from build123d import *

# Parameters (mm, degrees)
F0_R      = 19.05
F1_DEPTH  = 101.6
F2_R      = 16.672802
F3_DEPTH  = 101.6
F5_DEPTH  = 101.6
F7_DEPTH  = 101.6
F9_DEPTH  = 101.6
F11_DEPTH = 101.6


with BuildPart() as f1:
    # F0 (on Right) → F1 (new body)
    with BuildSketch(Plane.YZ):
        Circle(F0_R)
    extrude(amount=F1_DEPTH)

    # F2 (on face) → F3 (cut)
    with BuildSketch(Plane.YZ.offset(101.6)):
        Circle(F2_R)
    extrude(amount=-F3_DEPTH, mode=Mode.SUBTRACT)

    # F4 (on face) → F5 (join)
    with BuildSketch(Plane(origin=(0, 0, 0), x_dir=(0, -1, 0), z_dir=(-1, 0, 0))):
        with BuildLine():
            Line((0, 19.05), (2.557494, 18.877545))
            ThreePointArc((2.557494, 18.877545), (5.998328, 44.666261), (2.622403, 70.463553))
            Line((2.622403, 70.463553), (0, 70.597149))
            ThreePointArc((0, 70.597149), (4.50405, 44.823575), (0, 19.05))
        make_face()
    extrude(amount=-F5_DEPTH)

    # F6 (on face) → F7 (join)
    with BuildSketch(Plane.YZ.offset(101.6)):
        with BuildLine():
            Line((-1.23902, -71.141139), (1.281651, -71.141139))
            ThreePointArc((1.281651, -71.141139), (5.279028, -45.073988), (1.281651, -19.006837))
            Line((1.281651, -19.006837), (-1.612408, -18.98164))
            ThreePointArc((-1.612408, -18.98164), (3.484779, -45.026237), (-1.23902, -71.141139))
        make_face()
    extrude(amount=-F7_DEPTH)

    # F8 (on face) → F9 (join)
    with BuildSketch(Plane(origin=(0, 0, 0), x_dir=(0, -1, 0), z_dir=(-1, 0, 0))):
        with BuildLine():
            Line((18.974914, 0), (18.974914, -1.689716))
            ThreePointArc((18.974914, -1.689716), (45.881311, -5.978723), (72.88587, -2.358837))
            Line((72.88587, -2.358837), (72.733122, -0.475401))
            ThreePointArc((72.733122, -0.475401), (45.817013, -4.422211), (18.974914, 0))
        make_face()
    extrude(amount=-F9_DEPTH)

    # F10 (on face) → F11 (join)
    with BuildSketch(Plane.YZ.offset(101.6)):
        with BuildLine():
            ThreePointArc((19.039206, -0.641189), (45.322797, 2.394132), (71.440637, -1.836555))
            Line((71.440637, -1.836555), (71.576953, 0.641189))
            ThreePointArc((71.576953, 0.641189), (45.30808, 4.934439), (19.039206, 0.641189))
            Line((19.039206, 0.641189), (19.039206, -0.641189))
        make_face()
    extrude(amount=-F11_DEPTH)


solid = f1.part
Read the model definition and answer for the solid it produces. Units are mm, in the model's axes. Give positions to 0.01 mm unless a question says otherwise; leave off trailing zeros. Write each loop counter-clockwise with the first axis right and the second up, starting at its lowest first coordinate (ties: lowest second). Pieces come first, ordered by that corner, then holes. Notation, with made-up numbers: (28.25, 37) - (54.25, 37) arc R20 cw to (54.25, 50) - close; hole circle Ø2 at (28.5, 89.5). An arc over 180 degrees is marked (long way). Answer in a Markdown table with one row per item. Add a question column.
Item 1: Flat-ended cylindrical pins translate along their axes: P1, Ø4, axis at x = 23, y = 43.5, coming from the +Z side; P2, Ø4, axis at x = 90, y = 19.5, coming from the -Z side; P3, Ø1, axis at x = 61, z = 42.5, coming from the +Y side; P4, Ø20, axis at y = 0, z = 0, coming from the -X side. Find the tip coordinate at first contact, or state that the pin passes through.
Item 2: Determine the mould class of faces 1 (the face through (51.5, 45, 2.4)), 2 (the face through (101.6, -6, -16)), 3 (the face through (51.51, 3.48, -44.65)) for opening direction Z: pulls with the +Z half, pulls with the -Z half, needs draft (parallel to the pull), parting line crosses it, or undercut.
Item 3: Section B-B, the plane z = 42 is taken. Write down the section's boundary in (x, y).
Item 4: Section A-A, the plane x = 38 is taken. Write down the section's boundary in (y, z).
Item 5: Section C-C, the plane y = -60.5 is taken. Write down the section's boundary in (x, z), and give its area (3 significant figures).
Item 6: Find the intervals of material crossed by L1, parallel to Z at x = 31, y = 12; L2, parallel to Y at x = 54.5, z = -13; L3, parallel to Z at x = 43.5, y = -6.5, in increasing order.
Recorded:
| question | item | result |
|---|---|---|
| 1 | P1 | stops at z = 4.93 |
| 1 | P2 | stops at z = -7.53 |
| 1 | P3 | stops at y = -4.45 |
| 1 | P4 | passes through |
| 2 | face 1 | pulls with the -Z half |
| 2 | face 2 | needs draft |
| 2 | face 3 | undercut |
| 3 | outline | (0, -5.96) - (101.6, -5.96) - (101.6, -4.45) - (0, -4.45) - close |
| 4 | outline | (-72.89, -2.36) arc R93.86 ccw to (-18.97, -1.69) arc R19.05 ccw to (-1.61, -18.98) arc R71.71 cw to (-1.24, -71.14) - (1.28, -71.14) arc R86.99 ccw to (1.28, -19.01) arc R19.05 ccw to (19.04, -0.64) arc R96.32 cw to (71.44, -1.84) - (71.58, 0.64) arc R82.51 ccw to (19.04, 0.64) arc R19.05 ccw to (0, 19.05) arc R75.99 cw to (0, 70.6) - (-2.62, 70.46) arc R99.3 ccw to (-2.56, 18.88) arc R19.05 ccw to (-19.05, -0.02) arc R88.42 cw to (-72.73, -0.48) - close; hole circle Ø33.35 at (0, 0) |
| 5 | outline | (0, -5.02) - (101.6, -5.02) - (101.6, -3.33) - (0, -3.33) - close |
| 5 | area | 172 mm2 |
| 6 | L1 | z = -14.8 to -11.58, 11.58 to 14.8 |
| 6 | L2 | y = -13.92 to -10.44, 10.44 to 13.92 |
| 6 | L3 | z = -17.91 to -15.35, 15.35 to 17.91 |
